For this review, take the finished solid that the model builds, in its own axes (mm). A direction names the side the tool comes from. Give positions to 0.01 mm unless a question says otherwise; leave off trailing zeros. Loops run counter-clockwise (first coordinate to the right, second up) from the corner with the lowest first, then second, coordinate; pieces in that order, holes last. Notation, with made-up numbers: (44, 16) - (95, 16) arc R16 cw to (95, 37) - close; hole circle Ø5 at (54.25, -22.5). An arc over 180 degrees is marked (long way). Answer in a Markdown table with one row per item.
Autodesk Inventor part; units mm, degrees
ref_plane "YZ Plane" through (0, 0, 0) normal (1, 0, 0) x (0, 1, 0)
ref_plane "XZ Plane" through (0, 0, 0) normal (0, 1, 0) x (-1, 0, 0)
ref_plane "XY Plane" through (0, 0, 0) normal (0, 0, 1) x (1, 0, 0)
sketch "スケッチ1" plane through (0, 0, 0) normal (0, 0, 1) x (1, 0, 0)
  circle A0 centre (0, 0) radius 16.75 construction
  circle A1 centre (0, 0) radius 32.5
  circle A2 centre (0, 0) radius 27.6 construction
  circle A3 centre (27.6, 0) radius 1.6
  circle A4 centre (19.5161, 19.5161) radius 1.6
  circle A5 centre (0, 27.6) radius 1.6
  circle A6 centre (-19.5161, 19.5161) radius 1.6
  circle A7 centre (-27.6, 0) radius 1.6
  circle A8 centre (-19.5161, -19.5161) radius 1.6
  circle A9 centre (0, -27.6) radius 1.6
  circle A10 centre (19.5161, -19.5161) radius 1.6
  circle A11 centre (0, 0) radius 16.95
  dimension "d11" = 55.2
  dimension "d9" = 65
  dimension "d10" = 33.5
  dimension "d12" = 3.2
  dimension "d15" = 360
  dimension "d17" = 33.9
extrude "押し出し3" add sketch "スケッチ1" along normal blind 3
sketch "スケッチ3" plane through (0, 0, 3) normal (0, 0, 1) x (1, 0, 0)
  circle A0 centre (0, 0) radius 32.5
  circle A1 centre (0, 0) radius 20.5
  circle A2 centre (0, 0) radius 16.95
  circle A3 centre (0, 0) radius 20.5
  circle A4 centre (0, 0) radius 16.95
extrude "押し出し4" cut sketch "スケッチ3" against normal blind 0.1 contours A1
properties part number "軸受けワッシャB_ダブルスラスト用(厚さ2mm_ポケットあり_ジュラコン)" material "アセタール樹脂、黒"
1. We need section D-D, the plane x = -15. Give the boundary of the cut face in (y, z).
Values:
| item | result |
|---|---|
| outline | (-28.83, 0) - (-7.89, 0) - (-7.89, 2.9) - (-13.97, 2.9) - (-13.97, 3) - (-28.83, 3) - close; (7.89, 0) - (28.83, 0) - (28.83, 3) - (13.97, 3) - (13.97, 2.9) - (7.89, 2.9) - close |
2. Clearance check with flat-ended pins moving along their axes: pin 1 (1.9 mm diameter, centred on x = 19.52, y = 19.52, fed in from +Z); pin 2 (12 mm diameter, centred on x = 9.5, y = 10, fed in from +Z); pin 3 (1 mm diameter, centred on y = -3.5, z = 2.5, fed in from +X); pin 4 (1 mm diameter, centred on x = -17.5, z = 1.5, fed in from +Y). State where each tip first meets the part, or that it passes through.
Values:
| item | result |
|---|---|
| pin 1 | passes through |
| pin 2 | stops at z = 2.9 |
| pin 3 | stops at x = 32.36 |
| pin 4 | stops at y = 27.7 |
3. Wall thickness on line 1 (Y direction, x = 0, z = 0.65); line 2 (X direction, y = -29, z = 2.5); line 3 (X direction, y = 18.5, z = 0.3): over which ranges is each line inside the solid? List them lowest first. Write a range as [from, to].
Values:
| item | result |
|---|---|
| line 1 | y = [-32.5, -29.2], [-26, -16.95], [16.95, 26], [29.2, 32.5] |
| line 2 | x = [-14.67, -0.77], [0.77, 14.67] |
| line 3 | x = [-26.72, -20.75], [-18.28, 18.28], [20.75, 26.72] |
4. We need section C-C, the plane z = 2.3. Count the separate pieces of the cut face and the enclosed holes in it, and give its area (3 significant figures).
Values:
| item | result |
|---|---|
| separate pieces | 1 |
| enclosed holes | 9 |
| area | 2,350 mm^2 |
5. We need section A-A, the plane y = 0. Give the boundary of the cut face in (x, z), and give its area (3 significant figures).
Values:
| item | result |
|---|---|
| outline | (-32.5, 0) - (-29.2, 0) - (-29.2, 3) - (-32.5, 3) - close; (-26, 0) - (-16.95, 0) - (-16.95, 2.9) - (-20.5, 2.9) - (-20.5, 3) - (-26, 3) - close; (16.95, 0) - (26, 0) - (26, 3) - (20.5, 3) - (20.5, 2.9) - (16.95, 2.9) - close; (29.2, 0) - (32.5, 0) - (32.5, 3) - (29.2, 3) - close |
| area | 73.4 mm^2 |
6. For faces 1 (the face through (20.254, -18.097, 1.479)), 2 (the face through (-7.7, 15.3, 2.9)), list the 3-axis set-ups (+Z, -Z, +X, -X, +Y, -Y) from which the entire face can be reached by the end or side of a thin tool; tool diameter is ignored.
Values:
| item | result |
|---|---|
| face 1 | +Z, -Z |
| face 2 | +Z |
7. Mouldability with a two-part tool opening along Y and no side actions: class faces 3 (the face through (31, -9.76, 1.48)), 4 (the face through (14, -14, 0)), 5 (the face through (-20.786, -18.543, 1.479)) as released by +Y, released by -Y, zero draft, split by the parting line, or undercut.
Values:
| item | result |
|---|---|
| face 3 | split by the parting line |
| face 4 | zero draft |
| face 5 | undercut |
